The listing builds one solid part. Answer for the finished solid, in the listing's coordinates (mm). Give positions to 0.01 mm unless a question says otherwise; leave off trailing zeros. Write each loop counter-clockwise with the first axis right and the second up, starting at its lowest first coordinate (ties: lowest second). Pieces come first, ordered by that corner, then holes. Notation, with made-up numbers: (47.25, 37.5) - (74.25, 37.5) arc R24 ccw to (74.25, 53.5) - close; hole circle Ø8 at (44.5, 87). An arc over 180 degrees is marked (long way). Answer in a Markdown table with one row per item. Add a question column.
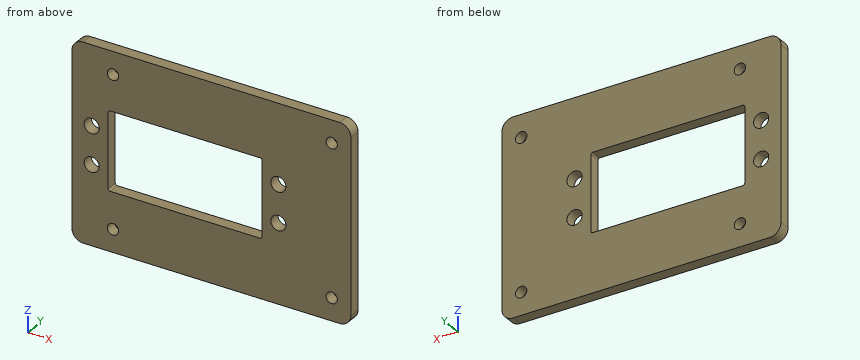
from build123d import *

# Parameters (mm, degrees)
SKETCH_1_W      = 60
SKETCH_1_H      = 52
SKETCH_1_R      = 2
SKETCH_1_R_2    = 1.5
SKETCH_1_W_2    = 40.8
SKETCH_1_H_2    = 20.8
SKETCH_1_W_3    = 14
EXTRUDE_1_DEPTH = 3
FILLET_1_R      = 0.5
FILLET_2_R      = 3


with BuildPart() as part:
    # 草图1 → 凸台-拉伸1 (new body)
    # profile 1 of 2: a face of its own
    with BuildSketch(Plane(origin=(0, 0, 0), x_dir=(1, 0, 0), z_dir=(0, 1, 0))):
        Rectangle(SKETCH_1_W, SKETCH_1_H)
        with Locations(Location((-24.75, 5, 0), (0, 0, 270))):
            Circle(SKETCH_1_R, mode=Mode.SUBTRACT)
        with Locations(Location((-24.75, -5, 0), (0, 0, 270))):
            Circle(SKETCH_1_R, mode=Mode.SUBTRACT)
        with Locations(Location((24.75, 5, 0), (0, 0, 270))):
            Circle(SKETCH_1_R, mode=Mode.SUBTRACT)
        with Locations(Location((24.75, -5, 0), (0, 0, 270))):
            Circle(SKETCH_1_R, mode=Mode.SUBTRACT)
        with Locations(Location((-19.11, 20, 0), (0, 0, 270))):
            Circle(SKETCH_1_R_2, mode=Mode.SUBTRACT)
        with Locations(Location((-19.11, -20, 0), (0, 0, 270))):
            Circle(SKETCH_1_R_2, mode=Mode.SUBTRACT)
        Rectangle(SKETCH_1_W_2, SKETCH_1_H_2, mode=Mode.SUBTRACT)
    # profile 2 of 2: a face of its own
    with BuildSketch(Plane(origin=(0, 0, 0), x_dir=(1, 0, 0), z_dir=(0, 1, 0))):
        with Locations((37, 0)):
            Rectangle(SKETCH_1_W_3, SKETCH_1_H)
        with Locations(Location((38.89, -20, 0), (0, 0, 270))):
            Circle(SKETCH_1_R_2, mode=Mode.SUBTRACT)
        with Locations(Location((38.89, 20, 0), (0, 0, 270))):
            Circle(SKETCH_1_R_2, mode=Mode.SUBTRACT)
    extrude(amount=EXTRUDE_1_DEPTH)

    # 圆角1
    fillet_1_edges = [part.edges().sort_by_distance(p)[0] for p in [
        (20.4, 1.5, -10.4),
        (-20.4, 1.5, -10.4),
        (-20.4, 1.5, 10.4),
        (20.4, 1.5, 10.4),
    ]]
    fillet(fillet_1_edges, radius=FILLET_1_R)

    # 圆角2
    fillet_2_edges = [part.edges().sort_by_distance(p)[0] for p in [
        (-30, 1.5, 26),
        (-30, 1.5, -26),
        (44, 1.5, -26),
        (44, 1.5, 26),
    ]]
    fillet(fillet_2_edges, radius=FILLET_2_R)


solid = part.part
1. Section D-D (z = -8) is taken. Give the vertices of the cut face in (x, y).
2. Straight lines are drawn through the part: L1, parallel to Z at x = -25, y = 0.5; L2, parallel to X at y = 2.75, z = -2.5; L3, parallel to X at y = 2.2, z = 5. For each, find the intervals that lie inside material, in ascending order. Write a range as [from, to].
3. Section C-C (x = -2) is taken. Give the vertices of the cut face in (y, z), and give its area (3 significant figures).
4. Given pin 1 Ø12 at (x, z) = (6.5, 0.5) entering from +Y, flat-ended and moving along its own axis, determine where the tip first touches the part or whether it passes through.
5. Section B-B (x = 24.75) is taken. Give the vertices of the cut face in (y, z), and give its area (3 significant figures).
6. Section A-A (z = 20) is taken. Give the vertices of the cut face in (x, y), and give its area (3 significant figures).
Geometry check:
| question | item | result |
|---|---|---|
| 1 | outline | (-30, 0) - (-20.4, 0) - (-20.4, 3) - (-30, 3) - close; (20.4, 0) - (44, 0) - (44, 3) - (20.4, 3) - close |
| 2 | L1 | [-26, -6.98], [-3.02, 3.02], [6.98, 26] |
| 2 | L2 | [-30, -20.4], [20.4, 44] |
| 2 | L3 | [-30, -26.75], [-22.75, -20.4], [20.4, 22.75], [26.75, 44] |
| 3 | outline | (0, -26) - (3, -26) - (3, -10.4) - (0, -10.4) - close; (0, 10.4) - (3, 10.4) - (3, 26) - (0, 26) - close |
| 3 | area | 93.6 mm² |
| 4 | pin 1 | through |
| 5 | outline | (0, -26) - (3, -26) - (3, -7) - (0, -7) - close; (0, -3) - (3, -3) - (3, 3) - (0, 3) - close; (0, 7) - (3, 7) - (3, 26) - (0, 26) - close |
| 5 | area | 132 mm² |
| 6 | outline | (-30, 0) - (-20.61, 0) - (-20.61, 3) - (-30, 3) - close; (-17.61, 0) - (37.39, 0) - (37.39, 3) - (-17.61, 3) - close; (40.39, 0) - (44, 0) - (44, 3) - (40.39, 3) - close |
| 6 | area | 204 mm² |
